Input: dimensioned drawing with shaded views. Units: mm. Origin: part minimum x, y, z. Coordinates: 2 decimals unless noted, no trailing zeros. Order: outer loops, then holes, each group sorted by start corner. A loop starts at its lowest first (then second) coordinate and runs counter-clockwise, first axis right, second up. Notation, with made-up numbers: (50.25, 25) -> (71.25, 25) arc R23 cw to (71.25, 51) -> close; hole circle Ø11 at (14.25, -38.75). An arc over 180 degrees is marked (long way). Put each result on its own line as item: value.
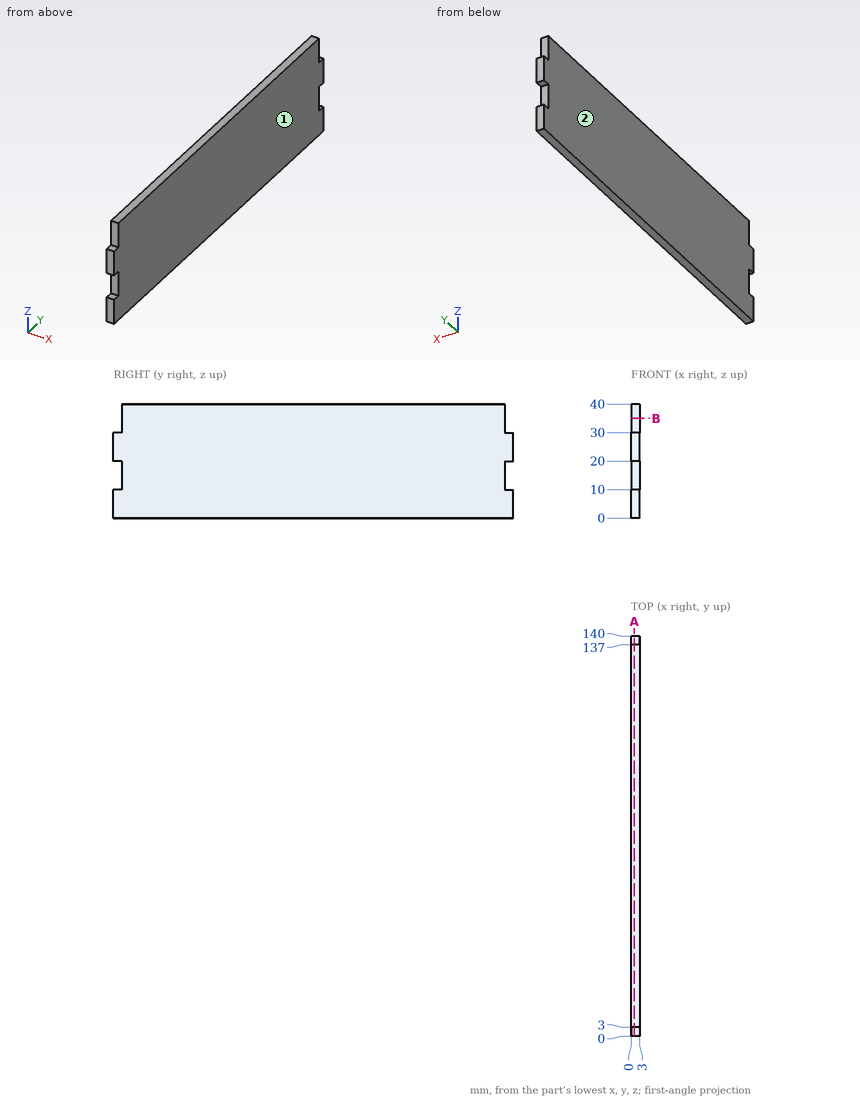
1. First-contact query: pin 1 (0.9 mm diameter, centred on x = 2, y = 1, fed in from +Z); pin 2 (1.5 mm diameter, centred on x = 1.5, z = 33, fed in from -Y); pin 3 (0.9 mm diameter, centred on x = 2, z = 17.5, fed in from +Y). Flat tips, straight axial feed; report the tip coordinate or a pass-through.
Numbers:
pin 1: stops at z = 30
pin 2: stops at y = 3
pin 3: stops at y = 137
2. Cut plane A-A on x = 1.1. Output: boundary loops of the cut face in (y, z).
Numbers:
outline: (0, 0) -> (140, 0) -> (140, 10) -> (137, 10) -> (137, 20) -> (140, 20) -> (140, 30) -> (137, 30) -> (137, 40) -> (3, 40) -> (3, 30) -> (0, 30) -> (0, 20) -> (3, 20) -> (3, 10) -> (0, 10) -> close
3. Cut plane B-B on z = 35. Output: boundary loops of the cut face in (x, y), plus the area to 3 significant figures.
Numbers:
outline: (0, 3) -> (3, 3) -> (3, 137) -> (0, 137) -> close
area: 402 mm2
4. Ray query, line 1 along Y through (x, z) = (2.8, 34.5). Return the intervals inside material, ascending.
Numbers:
line 1: y = 3 to 137
5. Pull-direction query (X, two-part tool) for the marked faces 1 and 2; classes: pulls with the +X half, pulls with the -X half, needs draft (parallel to the pull), parting line crosses it, or undercut.
Numbers:
face 1: pulls with the +X half
face 2: pulls with the -X half
